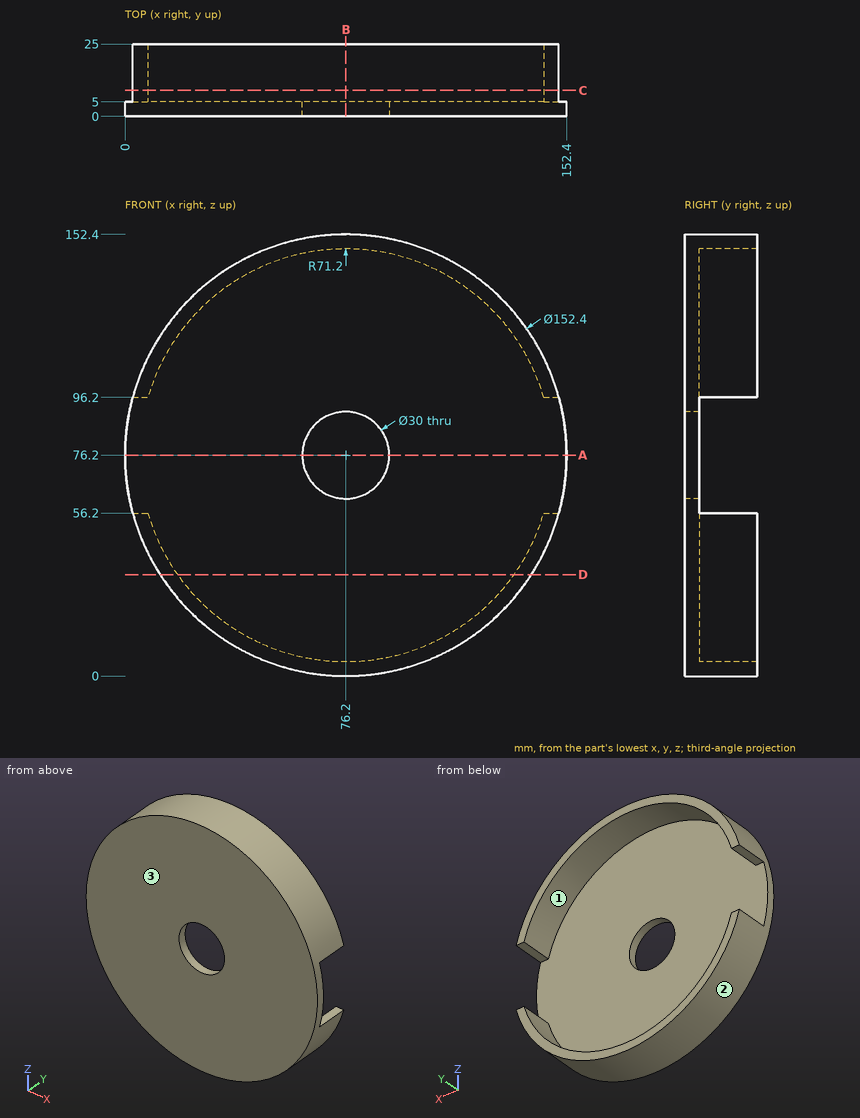
Could you check a few things on this drawing? It's one solid part, dimensions in mm from its lowest x, y, z. Round coordinates to 2 decimals unless told otherwise and drop trailing zeros. Write each loop counter-clockwise with the first axis right and the second up, starting at its lowest first coordinate (ties: lowest second). Pieces come first, ordered by that corner, then holes. Notation, with made-up numbers: (42, 81.25) -> (49, 81.25) arc R20 ccw to (49, 91.25) -> close; hole circle Ø6 at (23, -15.75). An arc over 180 degrees is marked (long way). One line per item, written item: value.
1) Suppose I cut it at B-B on x = 76.2. List the corners of the cut face in (y, z) for me.
Filled sheet:
outline: (0, 0) -> (25, 0) -> (25, 5) -> (5, 5) -> (5, 61.2) -> (0, 61.2) -> close; (0, 91.2) -> (5, 91.2) -> (5, 147.4) -> (25, 147.4) -> (25, 152.4) -> (0, 152.4) -> close
2) I'm going to push flat-ended pins straight in: pin 1 Ø12 at (x, y) = (135, 17.5) entering from -Z; pin 2 Ø18 at (x, z) = (76.2, 76.2) entering from -Y; pin 3 Ø1 at (x, y) = (20, 22.5) entering from -Z; pin 4 Ø4 at (x, z) = (34.5, 44.5) entering from +Y. Where does each tip first touch, or does it pass through?
Filled sheet:
pin 1: stops at z = 21.26
pin 2: passes through
pin 3: stops at z = 24.2
pin 4: stops at y = 5
3) Suppose I cut it at D-D on z = 35. List the corners of the cut face in (x, y) for me, plus the area to 3 significant figures.
Filled sheet:
outline: (12.1, 0) -> (140.3, 0) -> (140.3, 25) -> (134.27, 25) -> (134.27, 5) -> (18.13, 5) -> (18.13, 25) -> (12.1, 25) -> close
area: 882 mm2
4) Suppose I cut it at A-A on z = 76.2. List the corners of the cut face in (x, y) for me, plus the area to 3 significant figures.
Filled sheet:
outline: (0, 0) -> (61.2, 0) -> (61.2, 5) -> (0, 5) -> close; (91.2, 0) -> (152.4, 0) -> (152.4, 5) -> (91.2, 5) -> close
area: 612 mm2
5) If I drill on line 1 (Z direction, x = 76.2, y = 3.85); line 2 (Y direction, x = 72.5, z = 142), over which ranges is the centre line in solid material (lowest first)? Write a range as [from, to].
Filled sheet:
line 1: z = [0, 61.2], [91.2, 152.4]
line 2: y = [0, 5]
6) Suppose I cut it at C-C on y = 9. List the corners of the cut face in (x, z) for me.
Filled sheet:
outline: (2.67, 56.2) arc R76.2 ccw to (149.73, 56.2) -> (144.53, 56.2) arc R71.2 cw to (7.87, 56.2) -> close; (2.67, 96.2) -> (7.87, 96.2) arc R71.2 cw to (144.53, 96.2) -> (149.73, 96.2) arc R76.2 ccw to start
7) We'd pull the mould along X, two halves only. Please class the marked faces 1, 2 and 3: released by +X, released by -X, zero draft, split by the parting line, or undercut.
Filled sheet:
face 1: undercut
face 2: split by the parting line
face 3: zero draft
